Work out the finished part from the listing and answer in its coordinate system (mm). A direction names the side the tool comes from. Give positions to 0.01 mm unless a question says otherwise; leave off trailing zeros. Loops run counter-clockwise (first coordinate to the right, second up) from the corner with the lowest first, then second, coordinate; pieces in that order, holes last. Notation, with made-up numbers: M 84.5,60 L 121.5,60 A20 ccw 121.5,76 Z; hole C 22.25,0.5 d2. An arc over 180 degrees is marked long. Answer as a JSON object with one key per item and string values. Group by question number.
```python
from build123d import *

# Parameters (mm, degrees)
SKETCH1_R           = 10
SKETCH1_R_2         = 7.56
BOSS_EXTRUDE1_DEPTH = 2.5
BOSS_EXTRUDE2_DEPTH = 5
BOSS_EXTRUDE3_DEPTH = 5
CHAMFER1_SIZE       = 0.2


with BuildPart() as part:
    # Sketch1 → Boss-Extrude1 (new body, symmetric)
    with BuildSketch(Plane(origin=(0, 0, 0), x_dir=(1, 0, 0), z_dir=(0, 1, 0))):
        Circle(SKETCH1_R)
        Circle(SKETCH1_R_2, mode=Mode.SUBTRACT)
    extrude(amount=BOSS_EXTRUDE1_DEPTH, both=True)

    # Sketch2 → Boss-Extrude2 (add)
    with BuildSketch(Plane(origin=(0, 2.5, 0), x_dir=(1, 0, 0), z_dir=(0, 1, 0))):
        with BuildLine():
            Line((-4.118009228, -6.34), (4.118009228, -6.34))
            ThreePointArc((4.118009228, -6.34), (0, -7.56), (-4.118009228, -6.34))
        make_face()
        with BuildLine():
            Line((-4.118009228, 6.34), (4.118009228, 6.34))
            ThreePointArc((4.118009228, 6.34), (0, 7.56), (-4.118009228, 6.34))
        make_face()
    extrude(amount=-BOSS_EXTRUDE2_DEPTH)

    # Sketch3 → Boss-Extrude3 (add)
    with BuildSketch(Plane(origin=(0, 2.5, 0), x_dir=(1, 0, 0), z_dir=(0, 1, 0))):
        with BuildLine():
            Line((-6, -8), (-1.2, -11.6))
            ThreePointArc((-1.2, -11.6), (0, -12), (1.2, -11.6))
            Line((1.2, -11.6), (6, -8))
            ThreePointArc((6, -8), (0, -10), (-6, -8))
        make_face()
    extrude(amount=-BOSS_EXTRUDE3_DEPTH)

    # Chamfer1
    chamfer1_edges = [part.edges().sort_by_distance(p)[0] for p in [
        (-7.56, 2.5, 0),
        (-7.56, -2.5, 0),
        (0, 2.5, 6.34),
        (0, -2.5, 6.34),
        (0, 2.5, -6.34),
        (0, -2.5, -6.34),
        (0, -2.5, -10),
        (-3.6, 2.5, 9.8),
        (0, 2.5, 12),
        (3.6, 2.5, 9.8),
        (3.6, -2.5, 9.8),
        (0, -2.5, 12),
        (-3.6, -2.5, 9.8),
        (0, 2.5, -10),
        (7.56, -2.5, 0),
        (7.56, 2.5, 0),
    ]]
    chamfer(chamfer1_edges, length=CHAMFER1_SIZE)


solid = part.part
```
Item 1: Given pin 1 Ø1.5 at (x, y) = (-6.5, -2) entering from -Z; pin 2 Ø1.4 at (x, y) = (-1, -0.5) entering from -Z; pin 3 Ø2 at (x, y) = (7, -0.5) entering from +Z, each flat-ended and moving along its own axis, determine where each tip first touches the part or whether it passes through.
Item 2: For a pull along X with two mould halves and no side action, classify faces 1 (the flat face through (3.6, 0, 9.8)), 2 (the flat face through (1, -2.5, 7)), 3 (the cylindrical face through (7.56, -0.03, 0.11)) as pulls with the +X half, pulls with the -X half, needs draft (parallel to the pull), parting line crosses it, or undercut.
Item 3: A tool of negligible diameter and unlimited length cuts with its end or side. For faces 4 (the flat face through (0, 0, -6.34)), 5 (the cylindrical face through (0, 0, 12)), from which of +Z, -Z, +X, -X, +Y, -Y can it reach the whole face along a straight path? Write none if from no direction.
Item 4: A cutting plane is placed at A-A (y = 0.65). Determine the outline of the cut face in (x, z), and give its area (3 significant figures).
Item 5: A cutting plane is placed at B-B (z = 0). Determine the outline of the cut face in (x, y), and give its area (3 significant figures).
Item 6: A cutting plane is placed at C-C (x = 0). Determine the outline of the cut face in (y, z), and give its area (3 significant figures).
Item 7: A cutting plane is placed at D-D (z = 9.75). Determine the outline of the cut face in (x, y), and give its area (3 significant figures).
Item 8: Find the intervals of material crossed by probe 1 along Z at (x, y) = (-8, 1.1); probe 2 along X at (y, z) = (0.6, -0.25); probe 3 along Z at (x, y) = (-4.75, 0.5), in increasing order. Write a range as [from, to].
The answers:
{
 "1": {"pin 1": "stops at z = -8.18", "pin 2": "stops at z = -10", "pin 3": "stops at z = 8"},
 "2": {"face 1": "pulls with the +X half", "face 2": "needs draft", "face 3": "undercut"},
 "3": {"face 4": "+Y, -Y", "face 5": "+Z, +Y, -Y"},
 "4": {"outline": "M -6,8 A10 ccw long 6,8 L 1.2,11.6 A2 ccw -1.2,11.6 Z; hole M -4.12,-6.34 L 4.12,-6.34 A7.56 ccw 4.12,6.34 L -4.12,6.34 A7.56 ccw Z", "area": "158 mm^2"},
 "5": {"outline": "M -10,-2.3 L -9.8,-2.5 L -7.76,-2.5 L -7.56,-2.3 L -7.56,2.3 L -7.76,2.5 L -9.8,2.5 L -10,2.3 Z; M 7.56,-2.3 L 7.76,-2.5 L 9.8,-2.5 L 10,-2.3 L 10,2.3 L 9.8,2.5 L 7.76,2.5 L 7.56,2.3 Z", "area": "24.2 mm^2"},
 "6": {"outline": "M -2.5,-9.8 L -2.3,-10 L 2.3,-10 L 2.5,-9.8 L 2.5,-6.54 L 2.3,-6.34 L -2.3,-6.34 L -2.5,-6.54 Z; M -2.5,6.54 L -2.3,6.34 L 2.3,6.34 L 2.5,6.54 L 2.5,11.8 L 2.3,12 L -2.3,12 L -2.5,11.8 Z", "area": "46.4 mm^2"},
 "7": {"outline": "M -3.67,-2.3 L -3.33,-2.5 L 3.33,-2.5 L 3.67,-2.3 L 3.67,2.3 L 3.33,2.5 L -3.33,2.5 L -3.67,2.3 Z", "area": "36.5 mm^2"},
 "8": {"probe 1": "z = [-6, 6]", "probe 2": "x = [-10, -7.56], [7.56, 10]", "probe 3": "z = [-8.8, -5.88], [5.88, 8.94]"}
}
